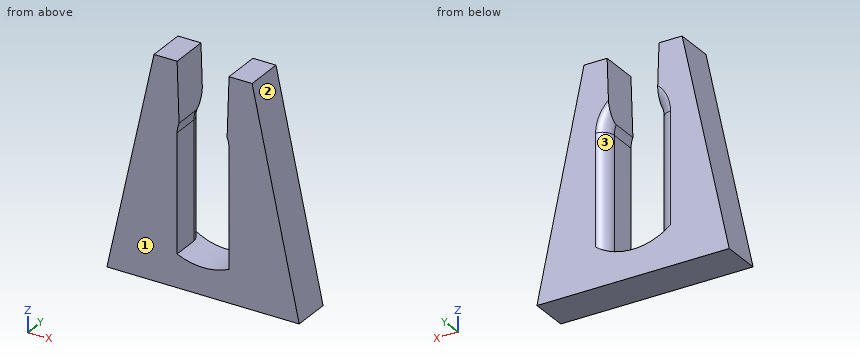
from build123d import *

# Parameters (mm, degrees)
PAD006_DEPTH = 10
FILLET001_R  = 3
PAD010_DEPTH = 4


with BuildPart() as part:
    # Sketch006 → Pad006 (new body)
    with BuildSketch(Plane.XZ):
        with BuildLine():
            Line((18.25, 57), (12.25, 57))
            Line((12.25, 57), (0, 0))
            Line((0, 0), (50, 0))
            Line((50, 0), (37.75, 57))
            Line((37.75, 57), (31.75, 57))
            Line((31.25, 41.54951), (31.75, 57))
            ThreePointArc((31.75, 39), (31.623821, 40.299038), (31.25, 41.54951))
            Line((31.749944, 8.5), (31.75, 39))
            ThreePointArc((18.249944, 8.5), (24.999944, 7), (31.749944, 8.5))
            Line((18.25, 39), (18.249944, 8.5))
            ThreePointArc((18.75, 41.54951), (18.376179, 40.299038), (18.25, 39))
            Line((18.75, 41.54951), (18.25, 57))
        make_face()
    extrude(amount=-PAD006_DEPTH)

    # Fillet001
    fillet001_edges = [part.edges().sort_by_distance(p)[0] for p in [
        (31.749972, 10, 23.75),
        (18.249972, 10, 23.75),
    ]]
    fillet(fillet001_edges, radius=FILLET001_R)

    # Sketch009 → Pad010 (join)
    with BuildSketch(Plane.XZ):
        Polygon((11, 6), (39, 6), (39, 0), (35, 0), (15, 0), (11, 0), align=None)
    extrude(amount=-PAD010_DEPTH)


solid = part.part
Read the model definition and answer for the solid it produces. Units are mm, in the model's axes. Face numbers are marked on the shaded views. Round coordinates to 2 decimals unless told otherwise and drop trailing zeros. Write each loop counter-clockwise with the first axis right and the second up, starting at its lowest first coordinate (ties: lowest second). Pieces come first, ordered by that corner, then holes. Notation, with made-up numbers: M 48,-4.75 L 105,-4.75 A7 cw 105,4.25 Z; hole C -12.75,86 d1. An arc over 180 degrees is marked long. Use a Markdown table: item, result.
1) The part is cut by section C-C (x = 39.5). Write down the section's boundary in (y, z).
Answers follow:
| item | result |
|---|---|
| outline | M 0,0 L 10,0 L 10,48.86 L 0,48.86 Z |
2) Straight lines are drawn through the part: line 1 along X through (y, z) = (1.25, 15); line 2 along X through (y, z) = (0.75, 31.5); line 3 along Z through (x, y) = (25, 9.25). For each, find the intervals that lie inside material, in ascending order. Write a range as [from, to].
Answers follow:
| item | result |
|---|---|
| line 1 | x = [3.22, 18.25], [31.75, 46.78] |
| line 2 | x = [6.77, 18.25], [31.75, 43.23] |
| line 3 | z = [0, 7] |
3) Flat-ended cylindrical pins translate along their axes: pin 1 (2 mm diameter, centred on x = 11, y = 7.5, fed in from -Z); pin 2 (1.5 mm diameter, centred on y = 5, z = 11.5, fed in from -X); pin 3 (2 mm diameter, centred on y = 5, z = 24.5, fed in from +X). Find the tip coordinate at first contact, or state that the pin passes through.
Answers follow:
| item | result |
|---|---|
| pin 1 | stops at z = 0 |
| pin 2 | stops at x = 2.31 |
| pin 3 | stops at x = 44.95 |
4) For a pull along Z with two mould halves and no side action, classify the marked faces 1, 2 and 3 as pulls with the +Z half, pulls with the -Z half, needs draft (parallel to the pull), parting line crosses it, or undercut.
Answers follow:
| item | result |
|---|---|
| face 1 | needs draft |
| face 2 | pulls with the +Z half |
| face 3 | undercut |
5) The part is cut by section A-A (z = 48.5). Write down the section's boundary in (x, y).
Answers follow:
| item | result |
|---|---|
| outline | M 10.42,0 L 18.53,0 L 18.53,10 L 10.42,10 Z; M 31.47,0 L 39.58,0 L 39.58,10 L 31.47,10 Z |
